For this review, take the finished solid that the model builds, in its own axes (mm). A direction names the side the tool comes from. Round coordinates to 2 decimals unless told otherwise and drop trailing zeros. Order: outer loops, then holes, each group sorted by start corner. A loop starts at its lowest first (then second) coordinate and runs counter-clockwise, first axis right, second up. Notation, with made-up numbers: M 11.25,-37.75 L 55.25,-37.75 A23 ccw 55.25,-16.75 Z; hole C -30.75,84 d6. An arc over 180 degrees is marked long. Answer as a JSON object with one key per item and string values.
from build123d import *

# Parameters (mm, degrees)
SKETCH1_W           = 281.317999974
SKETCH1_H           = 564.917999956
BOSS_EXTRUDE1_DEPTH = 2.640000816
SKETCH2_W           = 281.317999974
SKETCH2_H           = 564.917999956
SKETCH2_W_2         = 276.918000138
SKETCH2_H_2         = 560.51800012
BOSS_EXTRUDE2_DEPTH = 203.2
SKETCH3_W           = 319.417999974
SKETCH3_H           = 603.017999956
SKETCH3_W_2         = 281.317999974
SKETCH3_H_2         = 564.917999956
BOSS_EXTRUDE3_DEPTH = 2.2
SKETCH5_W           = 276.918000138
SKETCH5_H           = 2.199999918
BOSS_EXTRUDE5_DEPTH = 152.4
SKETCH7_R           = 3.175
BOSS_EXTRUDE6_DEPTH = 2.2
LPATTERN1_COUNT     = 6
LPATTERN1_PITCH     = 80.399999982
FILLET4_R           = 9.525


with BuildPart() as part:
    # Sketch1 → Boss-Extrude1 (new body)
    with BuildSketch(Plane(origin=(0, 0, 0), x_dir=(1, 0, 0), z_dir=(0, 1, 0))):
        Rectangle(SKETCH1_W, SKETCH1_H)
    extrude(amount=BOSS_EXTRUDE1_DEPTH)

    # Sketch2 → Boss-Extrude2 (add)
    with BuildSketch(Plane(origin=(0, 2.640000816, 0), x_dir=(1, 0, 0), z_dir=(0, 1, 0))):
        Rectangle(SKETCH2_W, SKETCH2_H)
        Rectangle(SKETCH2_W_2, SKETCH2_H_2, mode=Mode.SUBTRACT)
    extrude(amount=BOSS_EXTRUDE2_DEPTH)

    # Sketch3 → Boss-Extrude3 (add)
    with BuildSketch(Plane(origin=(0, 205.840000816, 0), x_dir=(1, 0, 0), z_dir=(0, 1, 0))):
        Rectangle(SKETCH3_W, SKETCH3_H)
        Rectangle(SKETCH3_W_2, SKETCH3_H_2, mode=Mode.SUBTRACT)
    extrude(amount=-BOSS_EXTRUDE3_DEPTH)

    # Sketch5 → Boss-Extrude5 (add)
    with BuildSketch(Plane(origin=(0, 2.640000816, 0), x_dir=(1, 0, 0), z_dir=(0, 1, 0))):
        with Locations((0, 200.959000037)):
            Rectangle(SKETCH5_W, SKETCH5_H)
    boss_extrude5 = extrude(amount=BOSS_EXTRUDE5_DEPTH)

    # Sketch7 → Boss-Extrude6 (add)
    # profile 1 of 2: a face of its own
    with BuildSketch(Plane.XY.offset(-199.859000078)):
        with BuildLine():
            Line((-79.525, 155.040000816), (-60.475, 155.040000816))
            Line((-60.475, 155.040000816), (-60.475, 177.265000816))
            ThreePointArc((-60.475, 177.265000816), (-70, 186.790000816), (-79.525, 177.265000816))
            Line((-79.525, 177.265000816), (-79.525, 155.040000816))
        make_face()
        with Locations((-70, 177.265000816)):
            Circle(SKETCH7_R, mode=Mode.SUBTRACT)
    # profile 2 of 2: a face of its own
    with BuildSketch(Plane.XY.offset(-199.859000078)):
        with BuildLine():
            Line((79.525, 155.040000816), (79.525, 177.265000816))
            ThreePointArc((79.525, 177.265000816), (70, 186.790000816), (60.475, 177.265000816))
            Line((60.475, 177.265000816), (60.475, 155.040000816))
            Line((60.475, 155.040000816), (79.525, 155.040000816))
        make_face()
        with Locations(Location((70, 177.265000816, 0), (0, 0, 180))):
            Circle(SKETCH7_R, mode=Mode.SUBTRACT)
    boss_extrude6 = extrude(amount=-BOSS_EXTRUDE6_DEPTH)

    # LPattern1: Boss-Extrude5, Boss-Extrude6 ×6
    with Locations(*[(0, 0, i * LPATTERN1_PITCH) for i in range(1, LPATTERN1_COUNT)]):
        add(boss_extrude5)
        add(boss_extrude6)

    # Fillet4
    fillet4_edges = [part.edges().sort_by_distance(p)[0] for p in [
        (-159.708999987, 204.740000816, -301.508999978),
        (159.708999987, 204.740000816, -301.508999978),
        (159.708999987, 204.740000816, 301.508999978),
        (-159.708999987, 204.740000816, 301.508999978),
    ]]
    fillet(fillet4_edges, radius=FILLET4_R)


solid = part.part
1) For L1, parallel to Y at x = -70, z = 201.65; L2, parallel to X at y = 158.5, z = 203.5; L3, parallel to Z at x = -123.5, y = 185.5, list the stretches that pass through material, from the lowest coordinate up.
Geometry check:
{"L1": "y = 0 to 174.09, 180.44 to 186.79", "L2": "x = -140.66 to -138.46, 138.46 to 140.66", "L3": "z = -282.46 to -280.26, 280.26 to 282.46"}
2) Insertion check: P1, Ø3, axis at x = -41.5, y = 183, coming from the -Z side; P2, Ø3, axis at x = 33, z = 210, coming from the +Y side; P3, Ø2, axis at x = 63.5, y = 143.5, coming from the +Z side; P4, Ø5, axis at x = -44.5, z = -215.5, coming from the -Y side. Each pin has a flat end and moves straight along its axis. Give the tip position at first contact, or say it passes through.
Geometry check:
{"P1": "stops at z = -282.46", "P2": "stops at y = 2.64", "P3": "stops at z = 282.46", "P4": "stops at y = 0"}
3) Mouldability with a two-part tool opening along X and no side actions: class faces 4 (the flat face through (-2, 100, -282.459)), 5 (the flat face through (-2, 93, 199.941)), 6 (the flat face through (-138.459, 103, 4)) as +X half, -X half, draft (parallel to the pull), parting line (faces both ways), or undercut.
Geometry check:
{"face 4": "draft", "face 5": "undercut", "face 6": "undercut"}
4) Add section B-B on z = 171. State the section outline as (x, y) points, and give its area (3 significant figures).
Geometry check:
{"outline": "M -159.71,203.64 L -140.66,203.64 L -140.66,0 L 140.66,0 L 140.66,203.64 L 159.71,203.64 L 159.71,205.84 L 138.46,205.84 L 138.46,2.64 L -138.46,2.64 L -138.46,205.84 L -159.71,205.84 Z", "area": "1,720 mm²"}
5) Add section A-A on y = 21. State how many separate pieces and enclosed holes the cut face has, and give its area (3 significant figures).
Geometry check:
{"separate pieces": "1", "enclosed holes": "7", "area": "7,360 mm²"}
6) Machinability: for faces 1 (the flat face through (-143, 203.64, -24)), 2 (the flat face through (-2, 0, -4)), 3 (the flat face through (-2, 93, 119.541)), which of the approach directions +Z, -Z, +X, -X, +Y, -Y give a long, thin tool a straight path to every point of the face, cutting with its end or side? Answer none if there is none.
Geometry check:
{"face 1": "-Y", "face 2": "+Z, -Z, +X, -X, -Y", "face 3": "+Y"}
